Geometry check sheet. Reference: the model listing, model coordinates, mm. A direction names the side the tool comes from. Round coordinates to 2 decimals unless told otherwise and drop trailing zeros. Order: outer loops, then holes, each group sorted by start corner. A loop starts at its lowest first (then second) coordinate and runs counter-clockwise, first axis right, second up. Notation, with made-up numbers: (40.25, 82.5) - (87.25, 82.5) arc R26 ccw to (87.25, 115.5) - close; hole circle Ø4 at (8, -34). An arc over 180 degrees is marked (long way). Use a Markdown table: item, result. Add a question column.
(1) Gauge pin test, flat ends, axial feed: P1, Ø1.1, axis at x = 9, z = 4.5, coming from the -Y side; P2, Ø1.3, axis at x = -8.5, z = 8, coming from the -Y side; P3, Ø0.6, axis at x = -7.5, z = 8.5, coming from the +Y side. Record the tip position at first contact, or that the pin passes through.
(2) Section check A-A on y = 11. Record the boundary of the cut face in (x, z).
(3) Access from +Z, -Z, +X, -X, +Y, -Y to the whole of each face (thin tool, end or side, straight path). Record for faces 1 (the face through (10.841, 16.822, 5.727)), 2 (the face through (-14.67, 8.59, 0.99)), 3 (the face through (-19.99, 0.98, 5.73)), 4 (the face through (20.005, 0.951, 5.727)).
(4) Mould release check, pull along X, two halves, no side actions. Record for faces 5 (the face through (10, 17, 11)), 6 (the face through (10.465, -15.874, 6.133)), 7 (the face through (-13.293, 16.046, 5.727)): released by +X, released by -X, zero draft, split by the parting line, or undercut.
(5) Thickness scan on line 1 along Y through (x, z) = (7.5, 1.5); line 2 along X through (y, z) = (17.5, 9.5); line 3 along Y through (x, z) = (-13.5, 1). Record the ranges inside material, lowest first. Write a range as [from, to].
(6) Section check D-D on y = 24.5. Record the boundary of the cut face in (x, z), then the cut area to 3 significant figures.
(7) Section check C-C on x = -13.5. Record the boundary of the cut face in (y, z).
(8) Section check B-B on z = 7.5. Give the number of separate pieces and of enclosed holes in the cut face, then the cut area to 3 significant figures.
```python
from build123d import *

# Parameters (mm, degrees)
BOSS_EXTRUDE1_DEPTH     = 1.4
SKETCH2_W               = 14.5
SKETCH2_H               = 10
BOSS_EXTRUDE2_DEPTH     = 0.6
BOSS_EXTRUDE3_DEPTH     = 11
BOSS_EXTRUDE4_DEPTH     = 0.6
CUT_EXTRUDE1_DEPTH      = 43.345719973
CUT_EXTRUDE1_DEPTH_BACK = 43.345719973


with BuildPart() as part:
    # Sketch1 → Boss-Extrude1 (new body)
    with BuildSketch(Plane.XY):
        Polygon((19.629909152, 0), (9.814954576, 17), (-9.814954576, 17), (-19.629909152, 0), (-9.814954576, -17), (9.814954576, -17), align=None)
    extrude(amount=BOSS_EXTRUDE1_DEPTH)

    # Sketch2 → Boss-Extrude2 (add)
    with BuildSketch(Plane.XY):
        with Locations((0, 22)):
            Rectangle(SKETCH2_W, SKETCH2_H)
        Polygon((19.757685902, 19.778684177), (27.007685902, 7.221315823), (18.347431864, 2.221315823), (11.097431864, 14.778684177), align=None)
        Polygon((27.007685902, -7.221315823), (19.757685902, -19.778684177), (11.097431864, -14.778684177), (18.347431864, -2.221315823), align=None)
        with Locations((0, -22)):
            Rectangle(SKETCH2_W, SKETCH2_H)
        Polygon((-19.757685902, -19.778684177), (-27.007685902, -7.221315823), (-18.347431864, -2.221315823), (-11.097431864, -14.778684177), align=None)
        Polygon((-27.007685902, 7.221315823), (-19.757685902, 19.778684177), (-11.097431864, 14.778684177), (-18.347431864, 2.221315823), align=None)
    extrude(amount=BOSS_EXTRUDE2_DEPTH)

    # Sketch3 → Boss-Extrude3 (add)
    with BuildSketch(Plane.XY):
        Polygon((-7.25, 22), (-8.05, 22), (-8.05, 17.8), (-10.276834792, 17.8), (-11.390252187, 15.8715045), (-15.027558883, 17.9715045), (-15.427558883, 17.278684177), (-11.097431864, 14.778684177), (-9.814954576, 17), (-7.25, 17), align=None)
        Polygon((15.427558883, 17.278684177), (15.027558883, 17.9715045), (11.390252187, 15.8715045), (10.276834792, 17.8), (8.05, 17.8), (8.05, 22), (7.25, 22), (7.25, 17), (9.814954576, 17), (11.097431864, 14.778684177), align=None)
        Polygon((22.677558883, -4.721315823), (23.077558883, -4.0284955), (19.440252187, -1.9284955), (20.553669583, 0), (19.440252187, 1.9284955), (23.077558883, 4.0284955), (22.677558883, 4.721315823), (18.347431864, 2.221315823), (19.629909152, 0), (18.347431864, -2.221315823), align=None)
        Polygon((7.25, -22), (8.05, -22), (8.05, -17.8), (10.276834792, -17.8), (11.390252187, -15.8715045), (15.027558883, -17.9715045), (15.427558883, -17.278684177), (11.097431864, -14.778684177), (9.814954576, -17), (7.25, -17), align=None)
        Polygon((-15.427558883, -17.278684177), (-15.027558883, -17.9715045), (-11.390252187, -15.8715045), (-10.276834792, -17.8), (-8.05, -17.8), (-8.05, -22), (-7.25, -22), (-7.25, -17), (-9.814954576, -17), (-11.097431864, -14.778684177), align=None)
        Polygon((-22.677558883, 4.721315823), (-23.077558883, 4.0284955), (-19.440252187, 1.9284955), (-20.553669583, 0), (-19.440252187, -1.9284955), (-23.077558883, -4.0284955), (-22.677558883, -4.721315823), (-18.347431864, -2.221315823), (-19.629909152, 0), (-18.347431864, 2.221315823), align=None)
    extrude(amount=BOSS_EXTRUDE3_DEPTH)

    # Sketch4 → Boss-Extrude4 (add)
    with BuildSketch(Plane.XY):
        Polygon((31.176914536, 0), (15.588457268, 27), (-15.588457268, 27), (-31.176914536, 0), (-15.588457268, -27), (15.588457268, -27), align=None)
    extrude(amount=BOSS_EXTRUDE4_DEPTH)

    # Sketch5 → Cut-Extrude1 (cut, two sides: drawn at the far end of the back side and taken through both)
    with BuildSketch(Plane.XY.offset(1.4).offset(-CUT_EXTRUDE1_DEPTH_BACK)):
        with BuildLine():
            Line((-5.5, 12), (5.5, 12))
            ThreePointArc((5.5, 12), (7.5, 10), (5.5, 8))
            Line((5.5, 8), (-5.5, 8))
            ThreePointArc((-5.5, 8), (-7.5, 10), (-5.5, 12))
        make_face()
    extrude(amount=CUT_EXTRUDE1_DEPTH + CUT_EXTRUDE1_DEPTH_BACK, mode=Mode.SUBTRACT)


solid = part.part
```
Check sheet entries:
| question | item | result |
|---|---|---|
| 1 | P1 | stops at y = -17.8 |
| 1 | P2 | stops at y = -22 |
| 1 | P3 | stops at y = 22 |
| 2 | outline | (-24.83, 0) - (-7.23, 0) - (-7.23, 1.4) - (-13.28, 1.4) - (-13.28, 0.6) - (-24.83, 0.6) - close; (7.23, 0) - (24.83, 0) - (24.83, 0.6) - (13.28, 0.6) - (13.28, 1.4) - (7.23, 1.4) - close |
| 3 | face 1 | +Z, +Y |
| 3 | face 2 | +Z |
| 3 | face 3 | +Z, -X |
| 3 | face 4 | +Z, +X |
| 4 | face 5 | zero draft |
| 4 | face 6 | undercut |
| 4 | face 7 | released by -X |
| 5 | line 1 | y = [-22, -17], [17, 22] |
| 5 | line 2 | x = [-15.3, -14.21], [-10.45, -7.25], [7.25, 10.45], [14.21, 15.3] |
| 5 | line 3 | y = [-17.09, -16.17], [-10.62, 10.62], [16.17, 17.09] |
| 6 | outline | (-17.03, 0) - (17.03, 0) - (17.03, 0.6) - (-17.03, 0.6) - close |
| 6 | area | 20.4 mm2 |
| 7 | outline | (-27, 0) - (27, 0) - (27, 0.6) - (17.09, 0.6) - (17.09, 11) - (16.17, 11) - (16.17, 0.6) - (10.62, 0.6) - (10.62, 1.4) - (-10.62, 1.4) - (-10.62, 0.6) - (-16.17, 0.6) - (-16.17, 11) - (-17.09, 11) - (-17.09, 0.6) - (-27, 0.6) - close |
| 8 | separate pieces | 6 |
| 8 | enclosed holes | 0 |
| 8 | area | 67.2 mm2 |
